For this review, take the finished solid that the model builds, in its own axes (mm). A direction names the side the tool comes from. Coordinates: 2 decimals unless noted, no trailing zeros. Loops run counter-clockwise (first coordinate to the right, second up) from the corner with the lowest first, then second, coordinate; pieces in that order, holes last. Notation, with made-up numbers: M 15.25,82 L 23.25,82 A26 ccw 23.25,116 Z; hole C 47,48.25 d4. An arc over 180 degrees is marked long. Use one line per item in the form item = value.
```python
from build123d import *

# Parameters (mm, degrees)
F1_DEPTH = 20
F2_W     = 13
F2_H     = 13
F3_DEPTH = 40
F4_R     = 2.5
F5_DEPTH = 14.813708499
F6_R     = 3


with BuildPart() as f1:
    # F0 (on Front) → F1 (new body)
    with BuildSketch(Plane.XZ):
        with BuildLine():
            Line((0, 10), (0, 0))
            Line((0, 0), (3, 0))
            ThreePointArc((3, 0), (6.5355339059, 1.4644660941), (8, 5))
            Line((8, 5), (8, 13))
            ThreePointArc((8, 13), (6.5355339059, 16.5355339059), (3, 18))
            Line((3, 18), (-11, 18))
            ThreePointArc((-11, 18), (-14.5355339059, 16.5355339059), (-16, 13))
            Line((-16, 13), (-16, 5.5269119346))
            ThreePointArc((-16, 5.5269119346), (-17.8519497029, 2.755273337), (-21.1213203436, 3.405591591))
            Line((-21.1213203436, 3.405591591), (-35.091883092, 17.3761543395))
            ThreePointArc((-35.091883092, 17.3761543395), (-37.2132034356, 18.2548339959), (-39.3345237792, 17.3761543395))
            Line((-39.3345237792, 17.3761543395), (-49.2340187158, 7.4766594029))
            ThreePointArc((-49.2340187158, 7.4766594029), (-50.1126983722, 5.3553390593), (-49.2340187158, 3.2340187158))
            Line((-49.2340187158, 3.2340187158), (-17.4644660941, -28.5355339059))
            ThreePointArc((-17.4644660941, -28.5355339059), (-16.3806023374, -30.15765065), (-16, -32.0710678119))
            Line((-16, -32.0710678119), (-16, -35))
            ThreePointArc((-16, -35), (-14.5355339059, -38.5355339059), (-11, -40))
            Line((-11, -40), (-8, -40))
            Line((-8, -40), (-8, 10))
            Line((-8, 10), (0, 10))
        make_face()
    extrude(amount=F1_DEPTH)

    # F2 (on face) → F3 (cut)
    with BuildSketch(Plane(origin=(-28.3553390593, 0, 28.3553390593), x_dir=(0, -1, 0), z_dir=(-0.7071067812, 0, 0.7071067812))):
        with Locations((10, -22.5269119346)):
            Rectangle(F2_W, F2_H)
    extrude(amount=-F3_DEPTH, mode=Mode.SUBTRACT)

    # F4 (on face) → F5 (cut, up to face)
    with BuildSketch(Plane(origin=(-0.0710678119, 0, 0.0710678119), x_dir=(0, -1, 0), z_dir=(-0.7071067812, 0, 0.7071067812))):
        with Locations((10, -22.5269119346)):
            Circle(F4_R)
    extrude(amount=-F5_DEPTH, mode=Mode.SUBTRACT)

    # F6
    f6_edges = [f1.edges().sort_by_distance(p)[0] for p in [
        (-44.284271, -20, 12.426407),
        (-44.284271, 0, 12.426407),
    ]]
    fillet(f6_edges, radius=F6_R)


solid = f1.part
```
1. Wall thickness on line 1 along Z through (x, y) = (-14, -10.75); line 2 along X through (y, z) = (-15.75, 1.5); line 3 along X through (y, z) = (-5.75, -32.5): over which ranges is each line inside the solid? List them lowest first. Write a range as from..to.
Computed values:
line_1 = -39..-21.23, -14.49..-13.86, -8.67..17
line_2 = -47.5..-42.55, -24.17..-8, 0..6.57
line_3 = -16..-8
2. For pin 1 Ø10 at (x, y) = (-30.5, -10) entering from +Z; pin 2 Ø2.5 at (x, y) = (-5.5, -7.5) entering from -Z; pin 3 Ø0.9 at (x, y) = (2, -12.5) entering from -Z; pin 4 Ø5 at (x, y) = (-39, -13) entering from +Z, all flat-tipped, find the tip position at first contact; note any pin that passes through.
Computed values:
pin_1 = 17.72
pin_2 = 10
pin_3 = 0
pin_4 = 18.25
3. Consider section C-C on y = -14.5. Write out the cut boundary in (x, z), plus the area to 3 significant figures.
Computed values:
outline = M -49.23,3.23 L -17.46,-28.54 A5 cw -16,-32.07 L -16,-35 A5 ccw -11,-40 L -8,-40 L -8,10 L 0,10 L 0,0 L 3,0 A5 ccw 8,5 L 8,13 A5 ccw 3,18 L -11,18 A5 ccw -16,13 L -16,5.53 A3 cw -21.12,3.41 L -35.09,17.38 A3 ccw -39.33,17.38 L -39.69,17.02 L -11.4,-11.26 L -20.6,-20.45 L -48.88,7.83 L -49.23,7.48 A3 ccw Z
area = 938 mm2
4. Tool access review of faces 1 (the face through (-4, -10, 18)), 2 (the face through (-28.009, -9.902, 10.293)), 3 (the face through (-4.1, -19.14, 17.1)), 4 (the face through (-15.1, -0.86, -33.56)): name each direction out of +Z, -Z, +X, -X, +Y, -Y from which nothing blocks a thin tool from reaching the whole face with its end or side.
Computed values:
face_1 = +Z, +X, +Y, -Y
face_2 = +Z, +Y, -Y
face_3 = +Z, +X, -Y
face_4 = -Z, -X, +Y
5. Consider section B-B on x = -6.5. Write out the cut boundary in (y, z), plus the area to 3 significant figures.
Computed values:
outline = M -20,10 L 0,10 L 0,15 A3 ccw -3,18 L -17,18 A3 ccw -20,15 Z
area = 156 mm2
6. Draft analysis for pull direction Z (two halves, no side actions). For faces 5 (the face through (-10, -10, -40)), 6 (the face through (8, -10, 9)), 7 (the face through (-25.744, -9.909, 3.078)), state which applies: +Z half, -Z half, draft (parallel to the pull), parting line (faces both ways), or undercut.
Computed values:
face_5 = -Z half
face_6 = draft
face_7 = undercut
7. Consider section A-A on z = -33. Write out the cut boundary in (x, y).
Computed values:
outline = M -16,-17 A3 ccw -13,-20 L -8,-20 L -8,0 L -13,0 A3 ccw -16,-3 Z
